from build123d import *

# Parameters (mm, degrees)
ESQUISSE1_W             = 364.4
ESQUISSE1_H             = 85
ESQUISSE1_W_2           = 300
ESQUISSE1_H_2           = 62.7
ESQUISSE1_H_3           = 37.7
BOSS_EXTRU_1_DEPTH      = 10
ESQUISSE3_R             = 2.25
ESQUISSE3_R_2           = 3
ENL_V_MAT_EXTRU_1_DEPTH = 10
ESQUISSE4_R             = 2.25
ENL_V_MAT_EXTRU_2_DEPTH = 10
CONG_1_R                = 10
CONG_2_R                = 2
ESQUISSE5_R             = 12.5
ENL_V_MAT_EXTRU_3_DEPTH = 10


with BuildPart() as part:
    # Esquisse1 → Boss.-Extru.1 (new body)
    with BuildSketch(Plane.XY):
        Rectangle(ESQUISSE1_W, ESQUISSE1_H)
        with Locations((0, 73.85)):
            Rectangle(ESQUISSE1_W_2, ESQUISSE1_H_2)
        Polygon((-150, 105.2), (-182.2, 42.5), (-150, 42.5), align=None)
        with Locations((0, -61.35)):
            Rectangle(ESQUISSE1_W_2, ESQUISSE1_H_3)
        Polygon((-150, -42.5), (-182.2, -42.5), (-150, -80.2), align=None)
        Polygon((182.2, 42.5), (150, 105.2), (150, 42.5), align=None)
        Polygon((182.2, -42.5), (150, -42.5), (150, -80.2), align=None)
    extrude(amount=BOSS_EXTRU_1_DEPTH)

    # Esquisse3 → Enlèv. mat.-Extru.1 (cut)
    with BuildSketch(Plane.XY.offset(10)):
        with Locations((-147.7, 32.5)):
            Circle(ESQUISSE3_R)
        with Locations((-172.2, 32.5)):
            Circle(ESQUISSE3_R_2)
        with Locations((-172.2, -32.5)):
            Circle(ESQUISSE3_R_2)
        with Locations((-147.7, -32.5)):
            Circle(ESQUISSE3_R)
        with Locations((172.2, -32.5)):
            Circle(ESQUISSE3_R_2)
        with Locations((147.7, -32.5)):
            Circle(ESQUISSE3_R)
        with Locations((172.2, 32.5)):
            Circle(ESQUISSE3_R_2)
        with Locations((147.7, 32.5)):
            Circle(ESQUISSE3_R)
    extrude(amount=-ENL_V_MAT_EXTRU_1_DEPTH, mode=Mode.SUBTRACT)

    # Esquisse4 → Enlèv. mat.-Extru.2 (cut)
    with BuildSketch(Plane.XY.offset(10)):
        with Locations((-122, -23.2)):
            Circle(ESQUISSE4_R)
        with Locations((122, -23.2)):
            Circle(ESQUISSE4_R)
    extrude(amount=-ENL_V_MAT_EXTRU_2_DEPTH, mode=Mode.SUBTRACT)

    # Congé1
    cong_1_edges = [part.edges().sort_by_distance(p)[0] for p in [
        (-150, -80.2, 5),
        (-150, 105.2, 5),
        (150, 105.2, 5),
        (150, -80.2, 5),
    ]]
    fillet(cong_1_edges, radius=CONG_1_R)

    # Congé2
    cong_2_edges = [part.edges().sort_by_distance(p)[0] for p in [
        (-182.2, -42.5, 5),
        (-182.2, 42.5, 5),
        (182.2, 42.5, 5),
        (182.2, -42.5, 5),
    ]]
    fillet(cong_2_edges, radius=CONG_2_R)

    # Esquisse5 → Enlèv. mat.-Extru.3 (cut)
    with BuildSketch(Plane(origin=(0, 0, 0), x_dir=(-1, 0, 0), z_dir=(0, 0, -1))):
        with Locations((92.2, -44.2)):
            Circle(ESQUISSE5_R)
    extrude(amount=-ENL_V_MAT_EXTRU_3_DEPTH, mode=Mode.SUBTRACT)


solid = part.part
CAD build for the part. Positions are in the model's coordinates, mm. Coordinates: 2 decimals unless noted, no trailing zeros. Order: outer loops, then holes, each group sorted by start corner. A loop starts at its lowest first (then second) coordinate and runs counter-clockwise, first axis right, second up.
Item 1: Band-saw the part on A-A on x = -88. List the corners of the cut face in (y, z).
Check sheet entries:
outline: (-80.2, 0) - (-55.97, 0) - (-55.97, 10) - (-80.2, 10) - close; (-32.43, 0) - (105.2, 0) - (105.2, 10) - (-32.43, 10) - close
Item 2: Band-saw the part on B-B on z = 4.75. Give the number of separate pieces and of enclosed holes in the cut face, plus the area to 3 significant figures.
Check sheet entries:
separate pieces: 1
enclosed holes: 11
area: 63,600 mm2
Item 3: Band-saw the part on D-D on y = 58.5. List the corners of the cut face in (x, z), plus the area to 3 significant figures.
Check sheet entries:
outline: (-173.98, 0) - (173.98, 0) - (173.98, 10) - (-173.98, 10) - close
area: 3,480 mm2
Item 4: Two-plate mould, pull along Y, no slides. Class faces 1 (the face through (182.2, 0, 5)), 2 (the face through (-149.631, -79.256, 5.07)), 3 (the face through (-79.712, -43.65, 4.93)): +Y half, -Y half, draft (parallel to the pull), parting line (faces both ways), or undercut.
Check sheet entries:
face 1: draft
face 2: -Y half
face 3: undercut
Item 5: Band-saw the part on C-C on y = -60.5. List the corners of the cut face in (x, z).
Check sheet entries:
outline: (-166.83, 0) - (166.83, 0) - (166.83, 10) - (-166.83, 10) - close
Item 6: Pin check, flat tip, straight feed: pin 1 Ø4 at (x, y) = (147.7, 32.5) entering from +Z. Stop position of the tip, or through.
Check sheet entries:
pin 1: passes through
Item 7: Drill centre lines: L1, parallel to Y at x = 147.7, z = 3.25; L2, parallel to Y at x = 172.2, z = 8; L3, parallel to Y at x = -92.2, z = 4. Where is each one in solid material? Low to high.
Check sheet entries:
L1: y = -79.93 to -34.75, -30.25 to 30.25, 34.75 to 104.45
L2: y = -54.21 to -35.5, -29.5 to 29.5, 35.5 to 61.97
L3: y = -80.2 to -56.7, -31.7 to 105.2
